```python
from build123d import *

# Parameters (mm, degrees)
F1_DEPTH = 12
F2_DEPTH = 75
F3_R     = 7
F4_DEPTH = 25
F5_R     = 15
F6_DEPTH = 5


with BuildPart() as f1:
    # F0 (on Top) → F1 (new body)
    with BuildSketch(Plane.XY):
        with BuildLine():
            ThreePointArc((-27.6872290695, 28.8689685727), (-28.772246751, 27.7877278111), (-29.8150709224, 26.6657373026))
            Line((-29.8150709224, 26.6657373026), (-29.8579817649, -26.6176806827))
            ThreePointArc((-29.8579817649, -26.6176806827), (-28.8178231022, -27.7404591103), (-27.7354722388, -28.8226227067))
            ThreePointArc((-27.7354722388, -28.8226227067), (15.6617545385, -36.8063777731), (40, 0))
            ThreePointArc((40, 0), (15.6925274768, 36.7932681532), (-27.6872290695, 28.8689685727))
        make_face()
        with BuildLine():
            Line((-27.6872290695, 28.8689685727), (-29.8132965897, 28.8689685727))
            Line((-29.8132965897, 28.8689685727), (-29.8150709224, 26.6657373026))
            ThreePointArc((-29.8150709224, 26.6657373026), (-28.772246751, 27.7877278111), (-27.6872290695, 28.8689685727))
        make_face()
        with BuildLine():
            Line((-29.8150709224, 26.6657373026), (-29.8132965897, 28.8689685727))
            ThreePointArc((-29.8132965897, 28.8689685727), (-38.4675305191, 15.5723824691), (-41.5, 0))
            ThreePointArc((-41.5, 0), (-38.480058979, -15.5413982954), (-29.8597560976, -28.8209119529))
            Line((-29.8597560976, -28.8209119529), (-29.8579817649, -26.6176806827))
            ThreePointArc((-29.8579817649, -26.6176806827), (-39.9999870288, 0.0322132702), (-29.8150709224, 26.6657373026))
        make_face()
        with BuildLine():
            Line((-29.8579817649, -26.6176806827), (-29.8150709224, 26.6657373026))
            ThreePointArc((-29.8150709224, 26.6657373026), (-39.9999870288, 0.0322132702), (-29.8579817649, -26.6176806827))
        make_face()
        with BuildLine():
            Line((-29.8579817649, -26.6176806827), (-29.8597560976, -28.8209119529))
            Line((-29.8597560976, -28.8209119529), (-27.7354722388, -28.8226227067))
            ThreePointArc((-27.7354722388, -28.8226227067), (-28.8178231022, -27.7404591103), (-29.8579817649, -26.6176806827))
        make_face()
    extrude(amount=F1_DEPTH)

    # F0 (on Top) → F2 (join)
    with BuildSketch(Plane.XY):
        with BuildLine():
            Line((-29.8043321806, 40.0002894977), (-59, 40.0002894977))
            Line((-59, 40.0002894977), (-59, -39.9997105023))
            Line((-59, -39.9997105023), (-29.8687587419, -39.9997105023))
            Line((-29.8687587419, -39.9997105023), (-29.8597560976, -28.8209119529))
            ThreePointArc((-29.8597560976, -28.8209119529), (-38.480058979, -15.5413982954), (-41.5, 0))
            ThreePointArc((-41.5, 0), (-38.4675305191, 15.5723824691), (-29.8132965897, 28.8689685727))
            Line((-29.8132965897, 28.8689685727), (-29.8043321806, 40.0002894977))
        make_face()
    extrude(amount=F2_DEPTH)

    # F3 (on face) → F4 (cut)
    with BuildSketch(Plane.XY.offset(12)):
        Circle(F3_R)
    extrude(amount=-F4_DEPTH, mode=Mode.SUBTRACT)

    # F5 (on face) → F6 (cut)
    with BuildSketch(Plane(origin=(-59, 0, 0), x_dir=(0, -1, 0), z_dir=(-1, 0, 0))):
        with Locations((0, 38.75)):
            Circle(F5_R)
    extrude(amount=-F6_DEPTH, mode=Mode.SUBTRACT)

    # F7: F1 across plane


with BuildPart() as f1_1:
    add(f1.part)
    add(f1.part.mirror(Plane.XY))


solid = f1_1.part
```
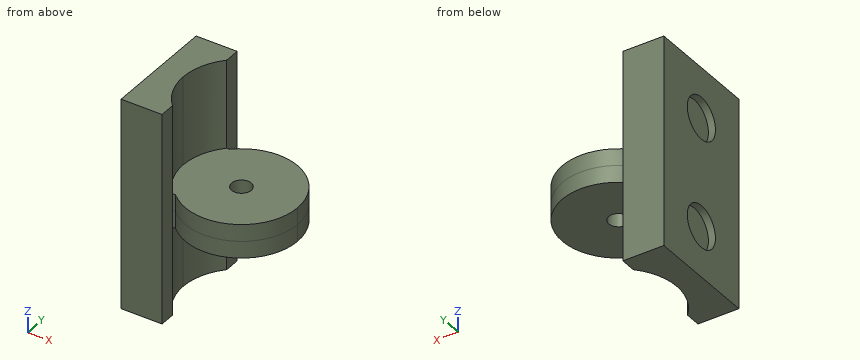
For this review, take the finished solid that the model builds, in its own axes (mm). Coordinates: 2 decimals unless noted, no trailing zeros. Loops run counter-clockwise (first coordinate to the right, second up) from the corner with the lowest first, then second, coordinate; pieces in that order, holes last.
1. Add section C-C, the plane y = -9. Give the boundary of the cut face in (x, z), then the cut area to 3 significant figures.
2. Add section B-B, the plane y = 35. Give the boundary of the cut face in (x, z), then the cut area to 3 significant figures.
3. Add section A-A, the plane z = 38.75. Give the boundary of the cut face in (x, y).
4. For line 1 (Z direction, x = -55, y = 0); line 2 (Y direction, x = 0, z = -8); line 3 (Z direction, x = -55, y = -6), list the stretches that pass through material, from the lowest coordinate up.
5. Add section D-D, the plane z = 16. Give the boundary of the cut face in (x, y).
6. Insertion check: P1, Ø5, axis at x = 26, z = 6, coming from the -Y side; P2, Ø8.5, axis at x = 0, y = 0, coming from the +Z side; P3, Ø10, axis at x = -9, y = -15.5, coming from the +Z side; P4, Ø8, axis at y = -10.5, z = -55, coming from the +X side. Each pin has a flat end and moves straight along its axis. Give the tip position at first contact, or say it passes through.
Result:
1. outline: (-59, -75) - (-40.51, -75) - (-40.51, -12) - (38.97, -12) - (38.97, 12) - (-40.51, 12) - (-40.51, 75) - (-59, 75) - (-59, 50.75) - (-54, 50.75) - (-54, 26.75) - (-59, 26.75) - (-59, -26.75) - (-54, -26.75) - (-54, -50.75) - (-59, -50.75) - close
1. area: 4,440 mm2
2. outline: (-59, -75) - (-29.81, -75) - (-29.81, 75) - (-59, 75) - close; (-19.36, -12) - (19.36, -12) - (19.36, 12) - (-19.36, 12) - close
2. area: 5,310 mm2
3. outline: (-59, -40) - (-29.87, -40) - (-29.86, -28.82) arc R41.5 cw to (-29.81, 28.87) - (-29.8, 40) - (-59, 40) - (-59, 15) - (-54, 15) - (-54, -15) - (-59, -15) - close
4. line 1: z = -75 to -53.75, -23.75 to 23.75, 53.75 to 75
4. line 2: y = -40 to -7, 7 to 40
4. line 3: z = -75 to -52.5, -25 to 25, 52.5 to 75
5. outline: (-59, -40) - (-29.87, -40) - (-29.86, -28.82) arc R41.5 cw to (-29.81, 28.87) - (-29.8, 40) - (-59, 40) - close
6. P1: stops at y = -32.37
6. P2: passes through
6. P3: stops at z = 12
6. P4: stops at x = -38.88
